Source: three-view drawing plus pictorial views. Frame: mm from the lowest corner of the part. A direction names the side the tool comes from. Give positions to 0.01 mm unless a question says otherwise; leave off trailing zeros. Order: outer loops, then holes, each group sorted by start corner. A loop starts at its lowest first (then second) coordinate and runs counter-clockwise, first axis right, second up. Notation, with made-up numbers: M 82,-12 L 121,-12 A15 cw 121,-4 Z; hole C 2.5,80 d7. An arc over 180 degrees is marked long. Use CSV: the item, a comma, the result in double quotes. Start each with the question number.
Item 1: Section query B-B on z = 35. Return loops of the section in (x, y).
Item 2: Ray query, probe 1 along Z at (x, y) = (40, 34); probe 2 along Z at (x, y) = (40, 32); probe 3 along X at (y, z) = (12.5, 25). Return the intervals inside material, ascending. Write a range as from..to.
Item 3: Pull-direction query (Z, two-part tool) for the marked faces 1, 2 and 3; classes: +Z half, -Z half, draft (parallel to the pull), parting line (faces both ways), or undercut.
Item 4: Section query C-C on x = 28. Return loops of the section in (y, z).
Item 5: Section query A-A on x = 40. Return loops of the section in (y, z), and give its area (3 significant figures).
Item 6: Access query for the marked faces 4 and 5. Directions: +Z, -Z, +X, -X, +Y, -Y. A direction counts if a zero-diameter tool reaches every point of the face in a straight line with its end or side. Return the directions, or none.
Item 7: Section query D-D on y = 5.5. Return loops of the section in (x, z), and give its area (3 significant figures).
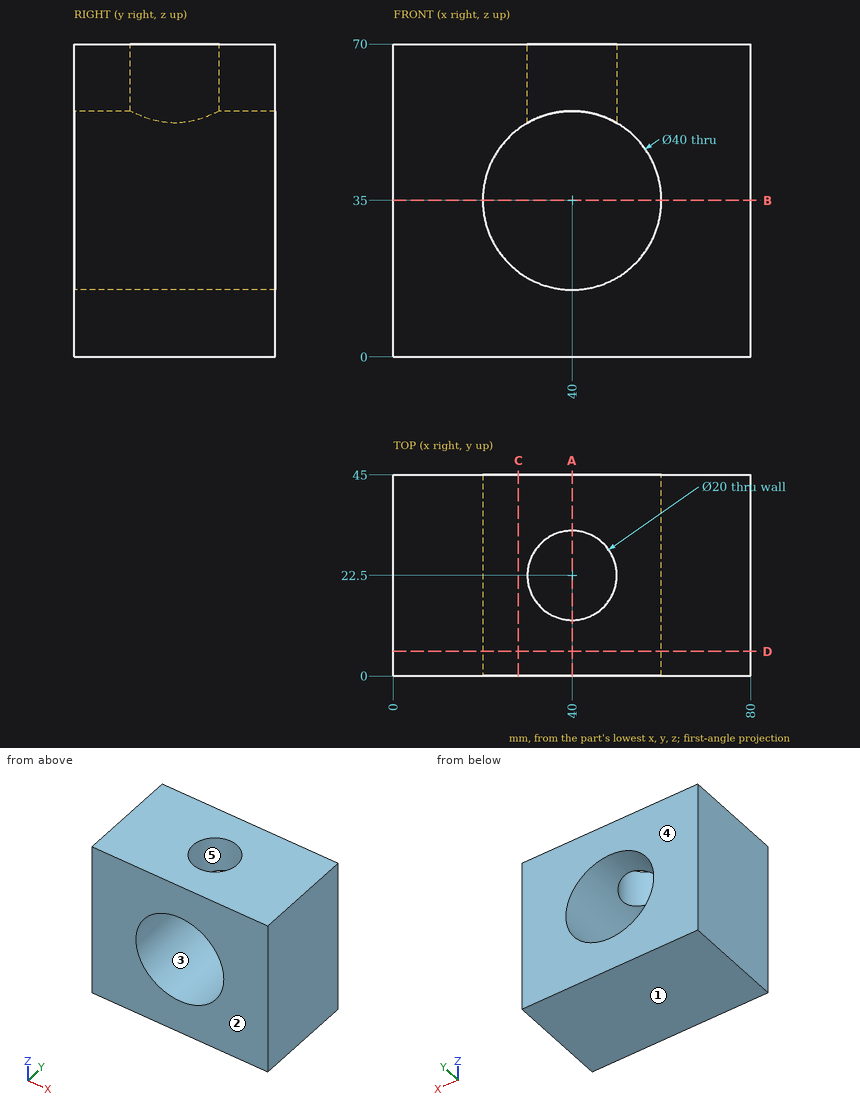
Verdict:
1,outline,"M 0,0 L 20,0 L 20,45 L 0,45 Z; M 60,0 L 80,0 L 80,45 L 60,45 Z"
2,probe 1,"0..15, 55..70"
2,probe 2,"0..15"
2,probe 3,"0..22.68, 57.32..80"
3,face 1,"-Z half"
3,face 2,"draft"
3,face 3,"undercut"
4,outline,"M 0,0 L 45,0 L 45,19 L 0,19 Z; M 0,51 L 45,51 L 45,70 L 0,70 Z"
5,outline,"M 0,0 L 45,0 L 45,15 L 0,15 Z; M 0,55 L 12.5,55 L 12.5,70 L 0,70 Z; M 32.5,55 L 45,55 L 45,70 L 32.5,70 Z"
5,area,"1,050 mm2"
6,face 4,"+Z, -Z, +X, -X, +Y"
6,face 5,"+Z"
7,outline,"M 0,0 L 80,0 L 80,70 L 0,70 Z; hole C 40,35 d40"
7,area,"4,340 mm2"
